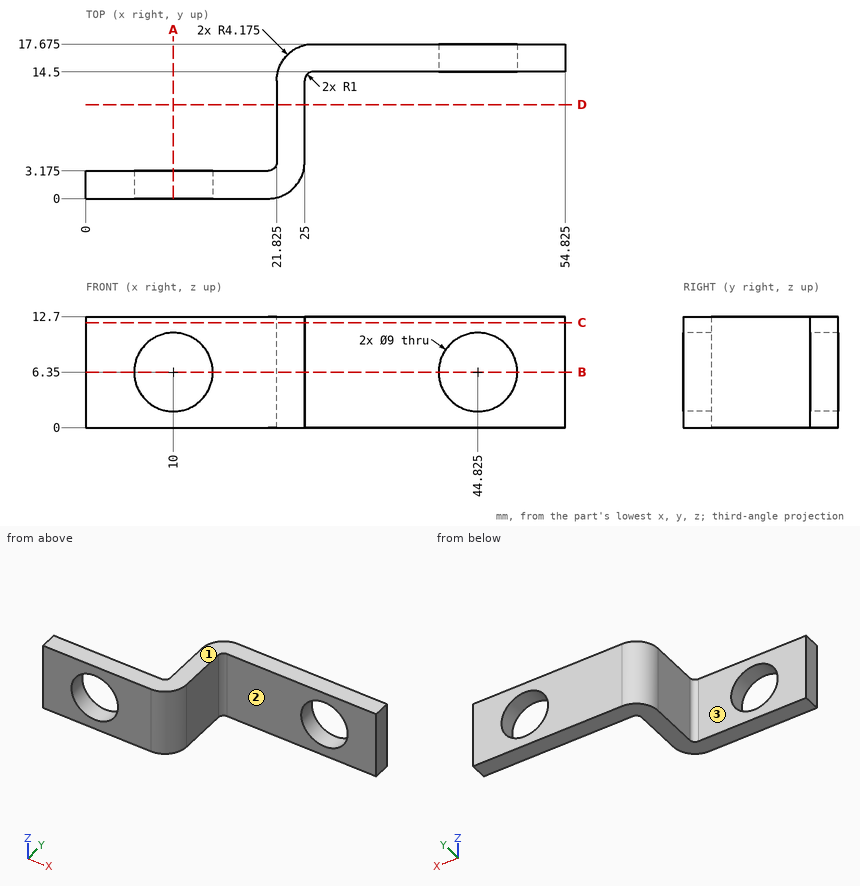
Design review of the part shown in the three views and the two pictorial views. Dimensions are in mm from the part's minimum x, y and z. A direction names the side the tool comes from. Round coordinates to 2 decimals unless told otherwise and drop trailing zeros. Write each loop counter-clockwise with the first axis right and the second up, starting at its lowest first coordinate (ties: lowest second). Pieces come first, ordered by that corner, then holes.
1) Take a section at C-C on z = 12. Give the boundary of the cut face in (x, y) (3 decimals).
Answer below:
outline: (0, 0) - (20.825, 0) arc R4.175 ccw to (25, 4.175) - (25, 13.5) arc R1 cw to (26, 14.5) - (54.825, 14.5) - (54.825, 17.675) - (26, 17.675) arc R4.175 ccw to (21.825, 13.5) - (21.825, 4.175) arc R1 cw to (20.825, 3.175) - (0, 3.175) - close
2) Take a section at A-A on x = 10. Give the boundary of the cut face in (y, z) (3 decimals), then the cut area to 3 significant figures.
Answer below:
outline: (0, 0) - (3.175, 0) - (3.175, 1.85) - (0, 1.85) - close; (0, 10.85) - (3.175, 10.85) - (3.175, 12.7) - (0, 12.7) - close
area: 11.7 mm2
3) Machinability: for the marked faces 1, 2 and 3, which of the approach directions +Z, -Z, +X, -X, +Y, -Y give a long, thin tool a straight path to every point of the face, cutting with its end or side? Answer none if there is none.
Answer below:
face 1: +Z, +X, -X, +Y, -Y
face 2: +Z, -Z, +X, -Y
face 3: +Z, -Z, -X, +Y
4) For line 1 along Y through (x, z) = (40, 11) (3 decimals); line 2 along Z through (x, y) = (10, 1.2); line 3 along Y through (x, z) = (18, 11) (3 decimals), list the stretches that pass through material, from the lowest coordinate up.
Answer below:
line 1: y = 14.5 to 17.675
line 2: z = 0 to 1.85, 10.85 to 12.7
line 3: y = 0 to 3.175
5) Insertion check: pin 1 Ø6 at (y, z) = (11, 9) entering from +X; pin 2 Ø4 at (y, z) = (8.5, 6) entering from +X; pin 3 Ø7.5 at (y, z) = (9.5, 6.5) entering from -X (3 decimals); pin 4 Ø1.5 at (x, y) = (31.5, 12.5) entering from +Z. Each pin has a flat end and moves straight along its axis. Give the tip position at first contact, or say it passes through.
Answer below:
pin 1: stops at x = 25.13
pin 2: stops at x = 25
pin 3: stops at x = 21.825
pin 4: passes through
6) Take a section at B-B on z = 6.35. Give the boundary of the cut face in (x, y) (3 decimals).
Answer below:
outline: (0, 0) - (5.5, 0) - (5.5, 3.175) - (0, 3.175) - close; (14.5, 0) - (20.825, 0) arc R4.175 ccw to (25, 4.175) - (25, 13.5) arc R1 cw to (26, 14.5) - (40.325, 14.5) - (40.325, 17.675) - (26, 17.675) arc R4.175 ccw to (21.825, 13.5) - (21.825, 4.175) arc R1 cw to (20.825, 3.175) - (14.5, 3.175) - close; (49.325, 14.5) - (54.825, 14.5) - (54.825, 17.675) - (49.325, 17.675) - close
7) Take a section at D-D on y = 10.75. Give the boundary of the cut face in (x, z) (3 decimals), then the cut area to 3 significant figures.
Answer below:
outline: (21.825, 0) - (25, 0) - (25, 12.7) - (21.825, 12.7) - close
area: 40.3 mm2
